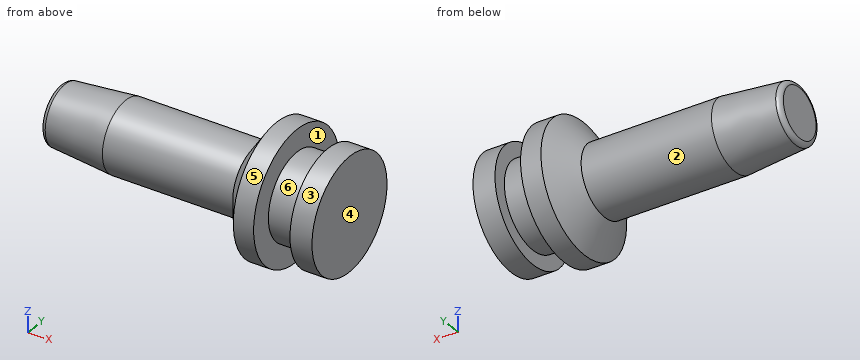
from build123d import *

# Parameters (mm, degrees)
FILETE1_R = 0.6


with BuildPart() as part:
    # Esboço1 → Revolução1 (revolve)
    with BuildSketch(Plane.XY, mode=Mode.PRIVATE) as revolu_o1_sk:
        Polygon((35.5, 0), (35.5, 7), (32.8, 7), (32.8, 5.25), (29, 5.25), (29, 8), (26.5, 8), (24, 4.3), (8, 4.3), (0, 3.6), (0, 0), align=None)
    revolve(revolu_o1_sk.sketch.rotate(Axis((0, 0, 0), (1, 0, 0)), 90), axis=Axis((0, 0, 0), (1, 0, 0)))

    # Filete1
    filete1_edges = [part.edges().sort_by_distance(p)[0] for p in [
        (0, 0, -3.6),
    ]]
    fillet(filete1_edges, radius=FILETE1_R)


solid = part.part
For this review, take the finished solid that the model builds, in its own axes (mm). Face numbers are marked on the shaded views. A direction names the side the tool comes from. Give positions to 0.01 mm unless a question says otherwise; leave off trailing zeros. Loops run counter-clockwise (first coordinate to the right, second up) from the corner with the lowest first, then second, coordinate; pieces in that order, holes last. Notation, with made-up numbers: M -16,5 L -4,5 A19 cw -4,12 Z; hole C 74.5,-17.5 d2. An arc over 180 degrees is marked long. Answer as a JSON object with one key per item and string values. Group by question number.
Q1. For probe 1 along X at (y, z) = (-1.5, -6); probe 2 along X at (y, z) = (-2, 5.25); probe 3 along Y at (x, z) = (34.5, -3), list the stretches that pass through material, from the lowest coordinate up. Write a range as [from, to].
Q2. Add section D-D on x = 26. Give the boundary of the cut face in (y, z), and give its area (3 significant figures).
Q3. Mouldability with a two-part tool opening along X and no side actions: class the marked faces 4, 5 and 6 as +X half, -X half, draft (parallel to the pull), parting line (faces both ways), or undercut.
Q4. Add section C-C on x = 10. Give the boundary of the cut face in (y, z), and give its area (3 significant figures).
Q5. Insertion check: P1, Ø4, axis at x = 32, z = 5.5, coming from the +Y side; P2, Ø3, axis at x = 30, y = -3, coming from the +Z side; P3, Ø3, axis at x = 4, y = 4, coming from the -Z side. Each pin has a flat end and moves straight along its axis. Give the tip position at first contact, or say it passes through.
Q6. Tool access review of the marked faces 1, 2 and 3: name each direction out of +Z, -Z, +X, -X, +Y, -Y from which nothing blocks a thin tool from reaching the whole face with its end or side.
Q7. Add section A-A on z = 0. Give the boundary of the cut face in (x, y).
Checked values:
{
 "1": {"probe 1": "[25.27, 29], [32.8, 35.5]", "probe 2": "[24.89, 29], [32.8, 35.5]", "probe 3": "[-6.32, 6.32]"},
 "2": {"outline": "C 0,0 d14.52", "area": "166 mm²"},
 "3": {"face 4": "+X half", "face 5": "draft", "face 6": "undercut"},
 "4": {"outline": "C 0,0 d8.6", "area": "58.1 mm²"},
 "5": {"P1": "y = 5.96", "P2": "z = 7.78", "P3": "z = -3.07"},
 "6": {"face 1": "none", "face 2": "-X", "face 3": "+X"},
 "7": {"outline": "M 0,-3.05 A0.6 ccw 0.55,-3.65 L 8,-4.3 L 24,-4.3 L 26.5,-8 L 29,-8 L 29,-5.25 L 32.8,-5.25 L 32.8,-7 L 35.5,-7 L 35.5,7 L 32.8,7 L 32.8,5.25 L 29,5.25 L 29,8 L 26.5,8 L 24,4.3 L 8,4.3 L 0.55,3.65 A0.6 ccw 0,3.05 Z"}
}
